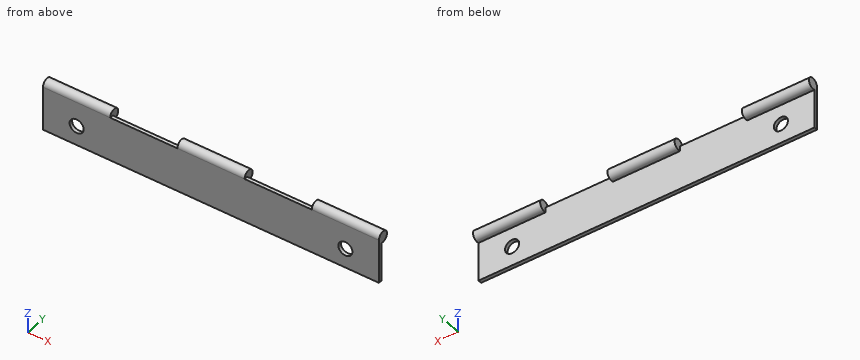
from build123d import *

# Parameters (mm, degrees)
SKETCH1_W               = 38.1
SKETCH1_H               = 12.7
BOSS_EXTRUDE1_DEPTH     = 1
SKETCH2_R               = 1.5875
BOSS_EXTRUDE2_DEPTH     = 19.05
MATRIZL1_COUNT          = 2
MATRIZL1_PITCH          = 38.1
SALIENTE_EXTRUIR1_DEPTH = 19.05
CROQUIS2_R              = 2
CORTAR_EXTRUIR1_DEPTH   = 19.05


with BuildPart() as part:
    # Sketch1 → Boss-Extrude1 (new body)
    with BuildSketch(Plane(origin=(0, 0, 0), x_dir=(1, 0, 0), z_dir=(0, 1, 0))):
        with Locations((19.05, 6.35)):
            Rectangle(SKETCH1_W, SKETCH1_H)
    boss_extrude1 = extrude(amount=BOSS_EXTRUDE1_DEPTH)

    # Sketch2 → Boss-Extrude2 (add)
    with BuildSketch(Plane.ZY):
        with Locations((0, 1.5875)):
            Circle(SKETCH2_R)
    boss_extrude2 = extrude(amount=-BOSS_EXTRUDE2_DEPTH)

    # MatrizL1: Boss-Extrude1, Boss-Extrude2 ×2
    with Locations(*[(i * MATRIZL1_PITCH, 0, 0) for i in range(1, MATRIZL1_COUNT)]):
        add(boss_extrude1)
        add(boss_extrude2)

    # Croquis1 → Saliente-Extruir1 (add)
    with BuildSketch(Plane(origin=(76.2, 0, 0), x_dir=(0, 0, -1), z_dir=(1, 0, 0))):
        with BuildLine():
            Line((12.7, 0), (0, 0))
            ThreePointArc((0, 0), (-0.890926484, 2.901427795), (1.47478812, 1))
            Line((1.47478812, 1), (12.7, 1))
            Line((12.7, 1), (12.7, 0))
        make_face()
    extrude(amount=SALIENTE_EXTRUIR1_DEPTH)

    # Croquis2 → Cortar-Extruir1 (cut)
    with BuildSketch(Plane(origin=(0, 1, 0), x_dir=(1, 0, 0), z_dir=(0, 1, 0))):
        with Locations(Location((85.725, 7.08739406, 0), (0, 0, 270))):
            Circle(CROQUIS2_R)
        with Locations(Location((9.525, 7.08739406, 0), (0, 0, 270))):
            Circle(CROQUIS2_R)
    extrude(amount=-CORTAR_EXTRUIR1_DEPTH, mode=Mode.SUBTRACT)


solid = part.part
Could you check a few things on this model? Use its own coordinates, in mm. Coordinates: 2 decimals unless noted, no trailing zeros. Order: outer loops, then holes, each group sorted by start corner. A loop starts at its lowest first (then second) coordinate and runs counter-clockwise, first axis right, second up. Notation, with made-up numbers: (75.25, -39) - (119.25, -39) arc R18 cw to (119.25, -4) - close; hole circle Ø7 at (5.5, 28.25). An arc over 180 degrees is marked (long way). Answer in a Markdown table with one row per item. Add a question column.
(1) If we section it at A-A, the plane y = 2.25: Please give me the cut outline in (x, z), then the cut area to 3 significant figures.
(2) Will these pins go through, and if not, where does the flat tip stop? pin 1 (1 mm diameter, centred on x = 85, z = -9.5, fed in from +Y); pin 2 (1.1 mm diameter, centred on x = 32.5, y = 0.5, fed in from +Z).
(3) If we section it at C-C, the plane x = 74: Please give me the cut outline in (y, z).
(4) I need wall thicknesses on L1, parallel to X at y = 2.15, z = -0.5; L2, parallel to X at y = 0.45, z = -7; L3, parallel to Z at x = 29, y = 0.7. Which ranges of each line are inside material? Lowest first, please.
(5) If we section it at B-B, the plane z = -4: Please give me the cut outline in (x, y).
Results are:
| question | item | result |
|---|---|---|
| 1 | outline | (0, -1.44) - (19.05, -1.44) - (19.05, 1.44) - (0, 1.44) - close; (38.1, -1.44) - (57.15, -1.44) - (57.15, 1.44) - (38.1, 1.44) - close; (76.2, -1.44) - (95.25, -1.44) - (95.25, 1.44) - (76.2, 1.44) - close |
| 1 | area | 165 mm2 |
| 2 | pin 1 | stops at y = 1 |
| 2 | pin 2 | stops at z = 0 |
| 3 | outline | (0, -12.7) - (1, -12.7) - (1, 0) - (0, 0) - close |
| 4 | L1 | x = 0 to 19.05, 38.1 to 57.15, 76.2 to 95.25 |
| 4 | L2 | x = 0 to 7.53, 11.52 to 83.73, 87.72 to 95.25 |
| 4 | L3 | z = -12.7 to 0 |
| 5 | outline | (0, 0) - (95.25, 0) - (95.25, 1) - (0, 1) - close |
